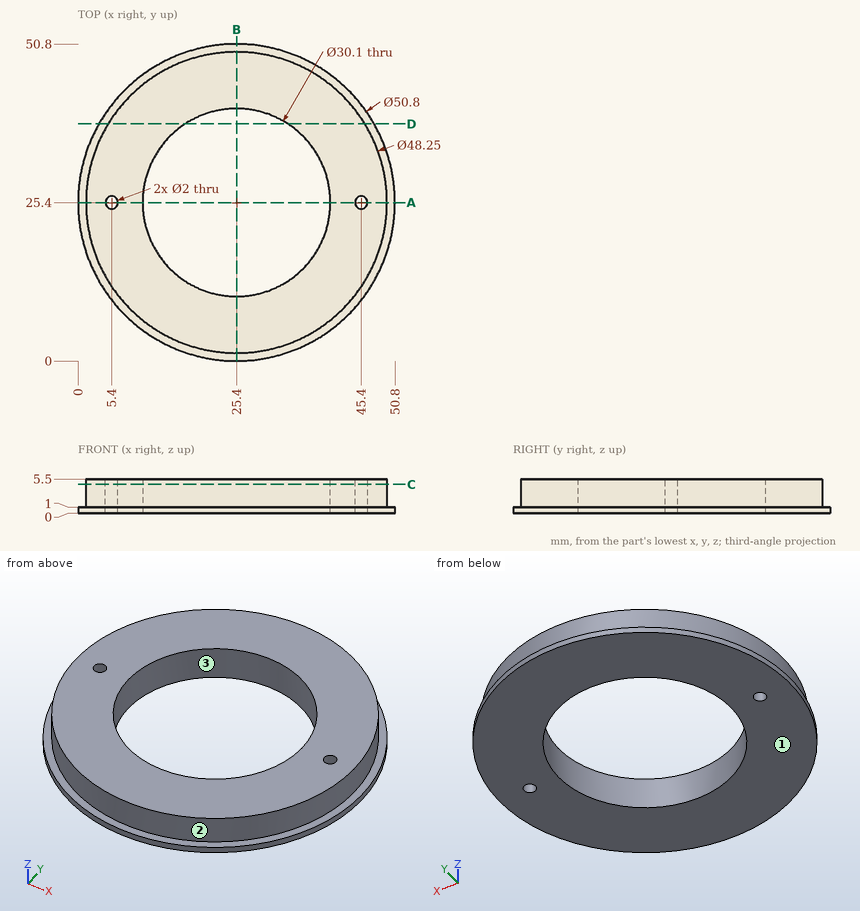
Geometry: see drawing. Coordinates: mm, zero at the bounding-box minimum. Give positions to 0.01 mm unless a question says otherwise; leave off trailing zeros. Order: outer loops, then holes, each group sorted by start corner. A loop starts at its lowest first (then second) coordinate and runs counter-clockwise, first axis right, second up. Notation, with made-up numbers: (35.25, -15.75) - (51.25, -15.75) arc R15 ccw to (51.25, -8.75) - close; hole circle Ø10 at (41, 28). An arc over 180 degrees is marked (long way). Write each question's results on one line, items separated by ' | '.
Item 1: Section D-D (y = 38). Return loops of the section in (x, z), and give its area (3 significant figures).
A:
outline: (3.35, 0) - (17.17, 0) - (17.17, 5.5) - (4.83, 5.5) - (4.83, 1) - (3.35, 1) - close; (33.63, 0) - (47.45, 0) - (47.45, 1) - (45.97, 1) - (45.97, 5.5) - (33.63, 5.5) - close | area: 139 mm^2
Item 2: Draft query along Y for the marked faces 1, 2 and 3. Return one class per face: released by +Y, released by -Y, zero draft, split by the parting line, or undercut.
A:
face 1: zero draft | face 2: split by the parting line | face 3: undercut
Item 3: Section C-C (z = 4.65). Return loops of the section in (x, y) (3 decimals).
A:
outline: circle Ø48.25 at (25.4, 25.4); hole circle Ø2 at (5.4, 25.4); hole circle Ø30.1 at (25.4, 25.4); hole circle Ø2 at (45.4, 25.4)
Item 4: Section B-B (x = 25.4). Return loops of the section in (y, z) (3 decimals).
A:
outline: (0, 0) - (10.35, 0) - (10.35, 5.5) - (1.275, 5.5) - (1.275, 1) - (0, 1) - close; (40.45, 0) - (50.8, 0) - (50.8, 1) - (49.525, 1) - (49.525, 5.5) - (40.45, 5.5) - close
Item 5: Material intervals for line 1 along Y through (x, z) = (25.4, 3.85) (3 decimals); line 2 along Y through (x, z) = (18, 1.8); line 3 along X through (y, z) = (37.5, 3.6), sorted ascending.
A:
line 1: y = 1.275 to 10.35, 40.45 to 49.525 | line 2: y = 2.44 to 12.29, 38.51 to 48.36 | line 3: x = 4.53 to 16.45, 34.35 to 46.27
Item 6: Contact query for flat-ended pins moving along their axis: pin 1 Ø3 at (x, z) = (43, 5) entering from -Y; pin 2 Ø1.5 at (y, z) = (8.5, 2) entering from -X; pin 3 Ø2 at (x, z) = (31, 2.5) entering from +Y. Output: stop coordinate, or through.
A:
pin 1: stops at y = 7.43 | pin 2: stops at x = 7.48 | pin 3: stops at y = 49.08
Item 7: Section A-A (y = 25.4). Return loops of the section in (x, z) (3 decimals).
A:
outline: (0, 0) - (4.4, 0) - (4.4, 5.5) - (1.275, 5.5) - (1.275, 1) - (0, 1) - close; (6.4, 0) - (10.35, 0) - (10.35, 5.5) - (6.4, 5.5) - close; (40.45, 0) - (44.4, 0) - (44.4, 5.5) - (40.45, 5.5) - close; (46.4, 0) - (50.8, 0) - (50.8, 1) - (49.525, 1) - (49.525, 5.5) - (46.4, 5.5) - close
